from build123d import *

# Parameters (mm, degrees)
F0_R     = 3.115166
F1_DEPTH = 12.7


with BuildPart() as f1:
    # F0 (on Top) → F1 (new body)
    with BuildSketch(Plane.XY):
        with BuildLine():
            ThreePointArc((-59.742244, -3.115166), (-59.327755, -1.58203), (-59.188154, 0))
            ThreePointArc((-59.188154, 0), (-59.642142, 2.827817), (-60.95848, 5.371418))
            ThreePointArc((-60.95848, 5.371418), (-77.164752, -1.281591), (-59.742244, -3.115166))
        make_face()
        with Locations((-68.222136, 0)):
            Circle(F0_R, mode=Mode.SUBTRACT)
        with BuildLine():
            ThreePointArc((-60.95848, 5.371418), (-59.642142, 2.827817), (-59.188154, 0))
            ThreePointArc((-59.188154, 0), (-59.327755, -1.58203), (-59.742244, -3.115166))
            Line((-59.742244, -3.115166), (66.04152, -3.115166))
            Line((66.04152, -3.115166), (66.04152, 5.371418))
            Line((66.04152, 5.371418), (-60.95848, 5.371418))
        make_face()
    extrude(amount=F1_DEPTH)


solid = f1.part
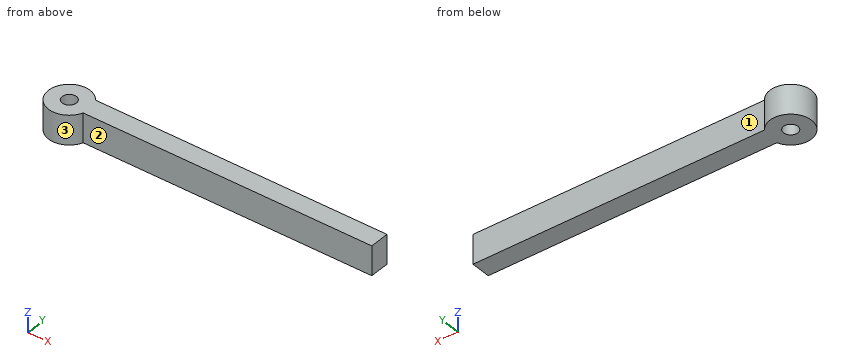
Check sheet for the modelled part. Datum: model origin and axes. Units: mm. Face numbers are marked on the shaded views. A direction names the side the tool comes from. Coordinates: 2 decimals unless noted, no trailing zeros. Write each loop counter-clockwise with the first axis right and the second up, starting at its lowest first coordinate (ties: lowest second). Pieces come first, ordered by that corner, then holes. Notation, with made-up numbers: M 64.5,49 L 119.5,49 A24 cw 119.5,77 Z; hole C 34.25,67.25 d8. An arc over 180 degrees is marked long. Answer as CSV lines item,"result".
Q1. Cross-section at A-A (y = 0). Record the boundary of the cut face in (x, z).
Check result:
outline,"M -77.26,0 L -71.34,0 L -71.34,12.7 L -77.26,12.7 Z; M -65.11,0 L 66.04,0 L 66.04,12.7 L -65.11,12.7 Z"
Q2. Cross-section at C-C (x = -39). Record the boundary of the cut face in (y, z).
Check result:
outline,"M -3.12,0 L 5.37,0 L 5.37,12.7 L -3.12,12.7 Z"
Q3. Go/stop test with flat-tipped pins: pin 1 (7 mm diameter, centred on x = -68.22, y = 0, fed in from +Z); pin 2 (5 mm diameter, centred on x = -43.5, z = 5, fed in from -Y); pin 3 (4 mm diameter, centred on y = -7, z = 11, fed in from -X); pin 4 (4 mm diameter, centred on x = 36.5, z = 11, fed in from +Y). Record where each tip stops, or that it passes through.
Check result:
pin 1,"z = 12.7"
pin 2,"y = -3.12"
pin 3,"x = -75.75"
pin 4,"y = 5.37"
Q4. Material ranges on probe 1 along Y at (x, z) = (-52.5, 2.25); probe 2 along X at (y, z) = (-2.25, 7.5); probe 3 along X at (y, z) = (-2.5, 10.5), recorded low to high. Write a range as from..to.
Check result:
probe 1,"-3.12..5.37"
probe 2,"-76.97..-70.38, -66.07..66.04"
probe 3,"-76.9..-70.08, -66.36..66.04"
Q5. Cross-section at B-B (z = 1.5). Record the boundary of the cut face in (x, y), then the cut area to 3 significant figures.
Check result:
outline,"M -60.96,5.37 A9.03 ccw long -59.74,-3.12 L 66.04,-3.12 L 66.04,5.37 Z; hole C -68.22,0 d6.23"
area,"1,290 mm^2"
Q6. Set-up check for the marked faces 1, 2 and 3: record each of +Z, -Z, +X, -X, +Y, -Y from which the full face is reachable in a straight line by a thin tool's end or side.
Check result:
face 1,"+Z, -Z, +X, +Y"
face 2,"+Z, -Z, +X, -Y"
face 3,"+Z, -Z"
Q7. Cross-section at D-D (y = -6.25). Record the boundary of the cut face in (x, z), then the cut area to 3 significant figures.
Check result:
outline,"M -74.75,0 L -61.7,0 L -61.7,12.7 L -74.75,12.7 Z"
area,"166 mm^2"
